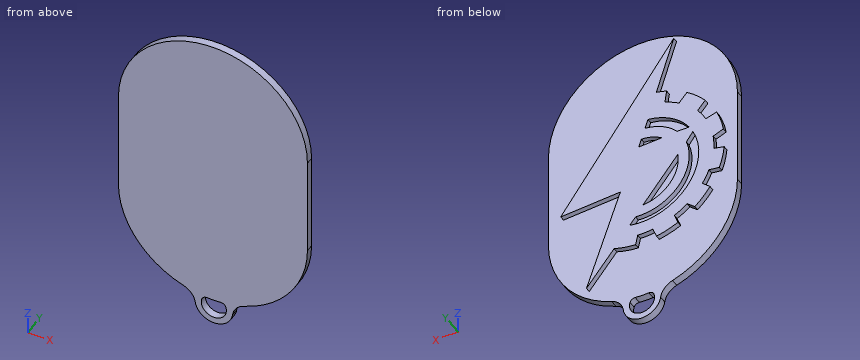
```python
from build123d import *

# Parameters (mm, degrees)
RESSALTO_EXTRUS_O1_DEPTH = 2
RESSALTO_EXTRUS_O2_DEPTH = 3
ESBO_O4_R                = 7.5
ESBO_O4_R_2              = 5
RESSALTO_EXTRUS_O3_DEPTH = 3
FILETE4_R                = 7
FILETE5_R                = 2


with BuildPart() as part:
    # Esboço1 → Ressalto-extrusão1 (new body)
    with BuildSketch(Plane(origin=(0, 0, 0), x_dir=(1, 0, 0), z_dir=(0, 1, 0))):
        with BuildLine():
            Line((35.368861757, 1.558526937), (80.44962534, 64.847807407))
            Line((80.44962534, 64.847807407), (56.661079085, 63.08569287))
            Line((56.661079085, 63.08569287), (70.170623872, 101.558526937))
            Line((70.170623872, 101.558526937), (59.156651238, 87.901974937))
            ThreePointArc((59.156651238, 87.901974937), (54.928228331, 89.016089828), (50.590505915, 89.568336625))
            Line((50.590505915, 89.568336625), (49.725051843, 85.574021555))
            ThreePointArc((49.725051843, 85.574021555), (46.713204504, 85.564588761), (43.718646065, 85.242202157))
            Line((43.718646065, 85.242202157), (42.238652592, 89.029169094))
            ThreePointArc((42.238652592, 89.029169094), (37.869771908, 87.87748691), (33.696266723, 86.146780478))
            Line((33.696266723, 86.146780478), (35.147163269, 82.442381585))
            ThreePointArc((35.147163269, 82.442381585), (32.519355747, 80.921668866), (30.065315343, 79.134037687))
            Line((30.065315343, 79.134037687), (26.950821583, 81.70865653))
            ThreePointArc((26.950821583, 81.70865653), (23.697250977, 78.547127541), (20.902055839, 74.973911711))
            Line((20.902055839, 74.973911711), (23.978190261, 72.338887308))
            ThreePointArc((23.978190261, 72.338887308), (22.53348512, 69.828267118), (21.346972592, 67.18581093))
            Line((21.346972592, 67.18581093), (17.203178516, 67.77029239))
            ThreePointArc((17.203178516, 67.77029239), (15.945727998, 63.496158243), (15.268245742, 59.09270252))
            Line((15.268245742, 59.09270252), (19.408088551, 58.19571674))
            ThreePointArc((19.408088551, 58.19571674), (19.397757282, 55.347323146), (19.667469692, 52.511708923))
            Line((19.667469692, 52.511708923), (15.579228762, 50.857655899))
            ThreePointArc((15.579228762, 50.857655899), (16.629849838, 46.377497076), (18.286206869, 42.084233852))
            Line((18.286206869, 42.084233852), (22.590276365, 43.394445807))
            ThreePointArc((22.590276365, 43.394445807), (24.103796918, 40.801148677), (25.877857628, 38.378620441))
            Line((25.877857628, 38.378620441), (22.860818156, 34.873071796))
            ThreePointArc((22.860818156, 34.873071796), (26.252016309, 31.352757541), (30.120648437, 28.365028835))
            Line((30.120648437, 28.365028835), (33.261631483, 31.944309078))
            ThreePointArc((33.261631483, 31.944309078), (36.017323235, 30.464825168), (38.916576083, 29.291350585))
            Line((38.916576083, 29.291350585), (38.221393853, 24.458284446))
            ThreePointArc((38.221393853, 24.458284446), (40.249791444, 23.869041331), (42.311374517, 23.409172359))
            Line((42.311374517, 23.409172359), (35.368861757, 1.558526937))
        make_face()
        with BuildLine():
            Line((45.69219136, 34.421477023), (46.852612972, 37.978627375))
            ThreePointArc((46.852612972, 37.978627375), (39.82616677, 40.034244908), (34.05073918, 44.533238778))
            Line((34.05073918, 44.533238778), (29.228152417, 44.533238778))
            ThreePointArc((29.228152417, 44.533238778), (36.346609181, 37.664247561), (45.69219136, 34.421477023))
        make_face(mode=Mode.SUBTRACT)
        with BuildLine():
            Line((48.310484351, 42.358641567), (49.345616552, 45.531730412))
            Line((49.345616552, 45.531730412), (40.18411035, 45.009645625))
            ThreePointArc((40.18411035, 45.009645625), (44.056709172, 43.099915587), (48.310484351, 42.358641567))
        make_face(mode=Mode.SUBTRACT)
        with BuildLine():
            Line((33.776854594, 55.159722076), (47.668932581, 72.651374716))
            ThreePointArc((47.668932581, 72.651374716), (36.882518839, 66.95561957), (33.776854594, 55.159722076))
        make_face(mode=Mode.SUBTRACT)
        with BuildLine():
            Line((30.333100839, 50.857655899), (27.743535352, 47.116522773))
            ThreePointArc((27.743535352, 47.116522773), (30.159670342, 71.285374829), (52.90625945, 79.803813767))
            Line((52.90625945, 79.803813767), (50.5964095, 76.848744643))
            ThreePointArc((50.5964095, 76.848744643), (33.326207959, 69.418591815), (30.333100839, 50.857655899))
        make_face(mode=Mode.SUBTRACT)
    extrude(amount=RESSALTO_EXTRUS_O1_DEPTH)

    # Esboço3 → Ressalto-extrusão2 (add)
    with BuildSketch(Plane.XZ):
        with BuildLine():
            Line((11.084172824, -74.126509554), (11.084172824, -34.266887476))
            ThreePointArc((11.084172824, -34.266887476), (48.761301795, 3.410241496), (86.438430767, -34.266887476))
            Line((86.438430767, -34.266887476), (86.438430767, -74.126509554))
            ThreePointArc((86.438430767, -74.126509554), (48.761301795, -111.803638526), (11.084172824, -74.126509554))
        make_face()
    extrude(amount=RESSALTO_EXTRUS_O2_DEPTH)

    # Esboço4 → Ressalto-extrusão3 (add)
    with BuildSketch(Plane(origin=(0, 0, 0), x_dir=(1, 0, 0), z_dir=(0, 1, 0))):
        with Locations((49.129422152, 114.56282345)):
            Circle(ESBO_O4_R)
        with Locations((49.129422152, 114.56282345)):
            Circle(ESBO_O4_R_2, mode=Mode.SUBTRACT)
    extrude(amount=-RESSALTO_EXTRUS_O3_DEPTH)

    # Filete4
    filete4_edges = [part.edges().sort_by_distance(p)[0] for p in [
        (42.394905756, -1.5, -111.261870721),
        (55.802725528, -1.5, -111.139809858),
    ]]
    fillet(filete4_edges, radius=FILETE4_R)

    # Filete5
    filete5_edges = [part.edges().sort_by_distance(p)[0] for p in [
        (45.084410441, -1.5, -111.623796356),
        (53.120255788, -1.5, -111.550640374),
    ]]
    fillet(filete5_edges, radius=FILETE5_R)


solid = part.part
```
Build history of the part. All positions in model axes, mm. Give positions to 0.01 mm unless a question says otherwise; leave off trailing zeros. Loops run counter-clockwise (first coordinate to the right, second up) from the corner with the lowest first, then second, coordinate; pieces in that order, holes last.
1) Drop flat-ended pins along their axis: P1, Ø2, axis at x = 53.5, y = -2, coming from the -Z side; P2, Ø1, axis at x = 44, y = 1, coming from the +Z side; P3, Ø1.6, axis at x = 31.5, y = 1.5, coming from the +Z side. Give the stop position or say it passes through.
Values follow:
P1: stops at z = -121.26
P2: stops at z = -12.97
P3: stops at z = -29.03
2) Probe line 1 along Y through (x, z) = (79, -83.5); line 2 along Z through (x, y) = (53.5, -2.8); line 3 along X through (y, z) = (1, -73.5). List the from-to ranges inside material, lowest first.
Values follow:
line 1: y = -3 to 0
line 2: z = -120.66 to -116.99, -112.36 to 3.11
line 3: x = 22.62 to 32.1, 37.66 to 60.32
3) Band-saw the part on B-B on z = -10. List the corners of the cut face in (x, y).
Values follow:
outline: (19.94, -3) - (77.58, -3) - (77.58, 0) - (41.38, 0) - (41.38, 2) - (38.05, 2) - (38.05, 0) - (19.94, 0) - close
4) Band-saw the part on A-A on x = 78. List the corners of the cut face in (y, z).
Values follow:
outline: (-3, -97.89) - (0, -97.89) - (0, -64.67) - (2, -64.67) - (2, -61.41) - (0, -61.41) - (0, -10.5) - (-3, -10.5) - close
5) Band-saw the part on C-C on z = -107.5. List the corners of the cut face in (x, y).
Values follow:
outline: (31.27, -3) - (66.25, -3) - (66.25, 0) - (31.27, 0) - close
